Verification items for the finished model (mm, model axes). A direction names the side the tool comes from. Round coordinates to 2 decimals unless told otherwise and drop trailing zeros. Order: outer loops, then holes, each group sorted by start corner. A loop starts at its lowest first (then second) coordinate and runs counter-clockwise, first axis right, second up. Notation, with made-up numbers: (51.25, 79.25) -> (70.25, 79.25) arc R26 cw to (70.25, 100.25) -> close; hole circle Ø6 at (66.25, 75). An arc over 180 degrees is marked (long way). Put each result on its own line as item: value.
from build123d import *

# Parameters (mm, degrees)
SKETCH_1_R      = 6
EXTRUDE_1_DEPTH = 120
SKETCH_2_W      = 12
SKETCH_2_H      = 5
CHAMFER_1_SIZE  = 0.5


with BuildPart() as part:
    # 草图1 → 凸台-拉伸1 (new body)
    with BuildSketch(Plane(origin=(0, 0, 0), x_dir=(1, 0, 0), z_dir=(0, 1, 0))):
        with Locations(Location((0, 0, 0), (0, 0, 270))):
            Circle(SKETCH_1_R)
    extrude(amount=EXTRUDE_1_DEPTH)

    # 草图2 → 旋转1 (revolve)
    with BuildSketch(Plane(origin=(0, 0, 0), x_dir=(0, 0, -1), z_dir=(1, 0, 0))):
        with Locations((6, 17.5)):
            Rectangle(SKETCH_2_W, SKETCH_2_H)
    revolve(axis=Axis((0, 0, 0), (0, 1, 0)))

    # 倒角1
    chamfer_1_edges = [part.edges().sort_by_distance(p)[0] for p in [
        (0, 0, -6),
        (0, 120, -6),
        (0, 20, 12),
        (0, 15, 12),
    ]]
    chamfer(chamfer_1_edges, length=CHAMFER_1_SIZE)


solid = part.part
Item 1: Section check A-A on x = 0. Record the boundary of the cut face in (y, z).
Check sheet entries:
outline: (0, -5.5) -> (0.5, -6) -> (15, -6) -> (15, -11.5) -> (15.5, -12) -> (19.5, -12) -> (20, -11.5) -> (20, -6) -> (119.5, -6) -> (120, -5.5) -> (120, 5.5) -> (119.5, 6) -> (20, 6) -> (20, 11.5) -> (19.5, 12) -> (15.5, 12) -> (15, 11.5) -> (15, 6) -> (0.5, 6) -> (0, 5.5) -> close
Item 2: Section check C-C on y = 36. Record the boundary of the cut face in (x, z).
Check sheet entries:
outline: circle Ø12 at (0, 0)
Item 3: Section check B-B on z = 0. Record the boundary of the cut face in (x, y), then the cut area to 3 significant figures.
Check sheet entries:
outline: (-12, 15.5) -> (-11.5, 15) -> (-6, 15) -> (-6, 0.5) -> (-5.5, 0) -> (5.5, 0) -> (6, 0.5) -> (6, 15) -> (11.5, 15) -> (12, 15.5) -> (12, 19.5) -> (11.5, 20) -> (6, 20) -> (6, 119.5) -> (5.5, 120) -> (-5.5, 120) -> (-6, 119.5) -> (-6, 20) -> (-11.5, 20) -> (-12, 19.5) -> close
area: 1,500 mm^2
Item 4: Material ranges on L1, parallel to Y at x = 0.5, z = -6.75; L2, parallel to X at y = 30.5, z = 0.25; L3, parallel to Z at x = -2.75, y = 45.5, recorded low to high. Write a range as [from, to].
Check sheet entries:
L1: y = [15, 20]
L2: x = [-5.99, 5.99]
L3: z = [-5.33, 5.33]
Item 5: Gauge pin test, flat ends, axial feed: pin 1 Ø1 at (x, z) = (-6.5, 1) entering from +Y; pin 2 Ø1 at (y, z) = (45.5, -0.5) entering from +X; pin 3 Ø4 at (y, z) = (62.5, 1.5) entering from -X; pin 4 Ø2 at (x, y) = (8.5, 96) entering from -Z. Record the tip position at first contact, or that the pin passes through.
Check sheet entries:
pin 1: stops at y = 20
pin 2: stops at x = 6
pin 3: stops at x = -6
pin 4: passes through
Item 6: Tool access check on faces 1 (the cylindrical face through (1.802, 7.648, 5.723)), 2 (the cylindrical face through (1.802, 69.054, 5.723)), 3 (the flat face through (0, 0, 0)). Record the directions out of +Z, -Z, +X, -X, +Y, -Y that give a thin tool (end or side, any length) a straight path to the whole face; none if there is none.
Check sheet entries:
face 1: -Y
face 2: +Y
face 3: +Z, -Z, +X, -X, -Y
